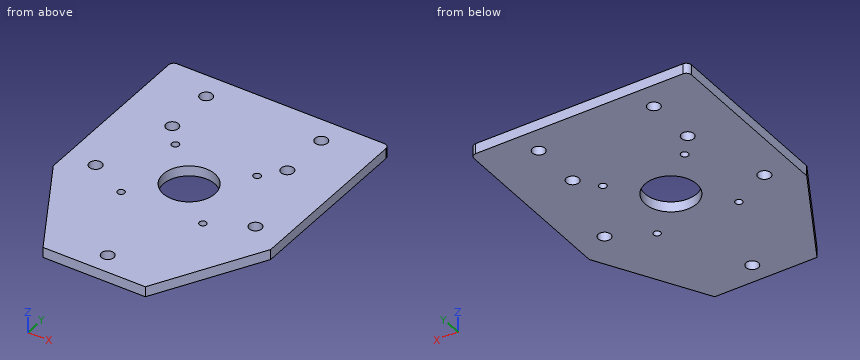
Autodesk Inventor part; units mm, degrees
ref_plane "YZ Plane" through (0, 0, 0) normal (1, 0, 0) x (0, 1, 0)
ref_plane "XZ Plane" through (0, 0, 0) normal (0, 1, 0) x (-1, 0, 0)
ref_plane "XY Plane" through (0, 0, 0) normal (0, 0, 1) x (1, 0, 0)
sketch "Sketch1" plane through (0, 0, 0) normal (0, 0, 1) x (1, 0, 0)
  line L0 (0, 0) -> (-20, 0)
  line L1 (-20, 0) -> (-42.5, 40)
  line L2 (-42.5, 40) -> (-42.5, 110)
  line L3 (-42.5, 110) -> (0, 110)
  circle A0 centre (0, 8) radius 2.45
  circle A1 centre (-31.25, 48) radius 2.45
  circle A2 centre (0, 56) radius 10.1211
  line L4 (16, 72) -> (-16, 72) construction
  line L5 (-16, 72) -> (-16, 40) construction
  line L6 (-16, 40) -> (16, 40) construction
  line L7 (16, 40) -> (16, 72) construction
  line L8 (16, 72) -> (-16, 40) construction
  line L9 (-16, 72) -> (16, 40) construction
  circle A3 centre (-16, 72) radius 1.45
  circle A4 centre (-16, 40) radius 1.4
  circle A5 centre (-22.5, 100) radius 2.45
  circle A6 centre (-22.5, 80) radius 2.45
  line L10 (0, 110) -> (0, 66.1211)
  line L11 (0, 45.8789) -> (0, 10.45)
  line L12 (0, 5.55) -> (0, 0)
  dimension "d0" = 20
  dimension "d2" = 40
  dimension "d3" = 70
  dimension "d4" = 4.9
  dimension "d5" = 4.9
  dimension "d6" = 32
  dimension "d7" = 32
  dimension "d8" = 8
  dimension "d9" = 40
  dimension "d10" = 8
  dimension "d11" = 2.9
  dimension "d12" = 2.8
  dimension "d13" = 4.9
  dimension "d14" = 4.9
  dimension "d15" = 10
  dimension "d16" = 30
  dimension "d17" = 20
  dimension "d18" = 20
extrude "Extrusion1" add sketch "Sketch1" along normal blind 4 contours L0 L1 L2 L3 L10 A2 L11 A0 L12
fillet "Fillet1" radius 2 1 edges at (-42.5, 110, 2)
mirror "Mirror1" about plane through (0, 66.1211, 0) normal (1, 0, 0) of "Extrusion1", "Fillet1"
ref_plane "Work Plane1" through (-20, 28, 0) normal (0, -1, 0) x (1, 0, 0)
equation "\"d17\" = d18"
properties part number "TOTEM_Base_Slide_x_20mmrod"
CAD build for the part. Positions are in the model's coordinates, mm. Round coordinates to 2 decimals unless told otherwise and drop trailing zeros. Order: outer loops, then holes, each group sorted by start corner. A loop starts at its lowest first (then second) coordinate and runs counter-clockwise, first axis right, second up.
Item 1: Saw through at D-D on x = -9. Write the cut outline in (y, z).
Item 2: Saw through at B-B on x = 0. Write the cut outline in (y, z).
Item 3: Saw through at A-A on y = 72. Write the cut outline in (x, z), then the cut area to 3 significant figures.
Item 4: Probe line 1 along X through (y, z) = (72, 1.5); line 2 along X through (y, z) = (56, 1.6); line 3 along Y through (x, z) = (31.25, 1.15). List the from-to ranges inside material, lowest first.
Item 5: Saw through at C-C on z = 1.05. State how many separate pieces and enclosed holes the cut face has, then the cut area to 3 significant figures.
Reported:
1. outline: (0, 0) - (51.37, 0) - (51.37, 4) - (0, 4) - close; (60.63, 0) - (110, 0) - (110, 4) - (60.63, 4) - close
2. outline: (0, 0) - (5.55, 0) - (5.55, 4) - (0, 4) - close; (10.45, 0) - (45.88, 0) - (45.88, 4) - (10.45, 4) - close; (66.12, 0) - (110, 0) - (110, 4) - (66.12, 4) - close
3. outline: (-42.5, 0) - (-17.45, 0) - (-17.45, 4) - (-42.5, 4) - close; (-14.55, 0) - (14.55, 0) - (14.55, 4) - (-14.55, 4) - close; (17.45, 0) - (42.5, 0) - (42.5, 4) - (17.45, 4) - close
3. area: 317 mm2
4. line 1: x = -42.5 to -17.45, -14.55 to 14.55, 17.45 to 42.5
4. line 2: x = -42.5 to -10.12, 10.12 to 42.5
4. line 3: y = 20 to 45.55, 50.45 to 110
5. separate pieces: 1
5. enclosed holes: 12
5. area: 7,970 mm2
